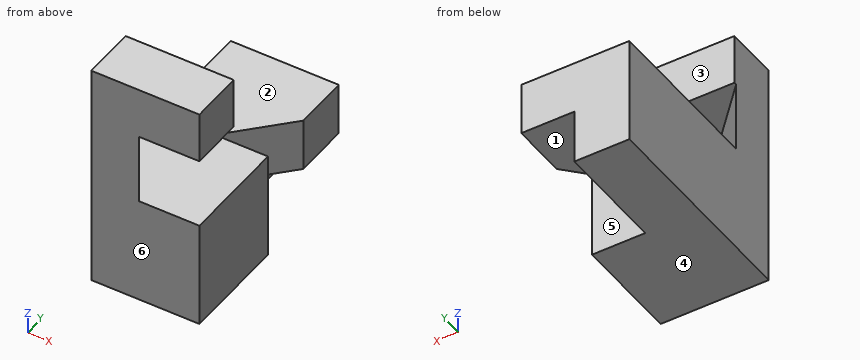
from build123d import *

# Parameters (mm, degrees)
F0_W      = 15.5
F0_H      = 15.5
F1_DEPTH  = 7.747
F3_DEPTH  = 10.16
F4_W      = 15.5
F4_H      = 7.75
F5_DEPTH  = 7.366
F6_W      = 7.874
F6_H      = 15.494
F7_DEPTH  = 16.002
F8_W      = 8.001
F8_H      = 7.62
F9_DEPTH  = 7.62
F11_DEPTH = 7.62


with BuildPart() as f1:
    # F0 (on Top) → F1 (new body, symmetric)
    with BuildSketch(Plane.XY):
        Rectangle(F0_W, F0_H)
    extrude(amount=F1_DEPTH, both=True)

    # F2 (on face) → F3 (join)
    with BuildSketch(Plane.XY.offset(7.747)):
        Polygon((-7.75, -0.384), (-7.75, -7.75), (-0.892, -7.75), align=None)
    extrude(amount=F3_DEPTH)

    # F4 (on face) → F5 (join)
    with BuildSketch(Plane.XY.offset(17.907)):
        with Locations((0, -3.875)):
            Rectangle(F4_W, F4_H)
    extrude(amount=F5_DEPTH)

    # F6 (on face) → F7 (join)
    with BuildSketch(Plane(origin=(0, 7.75, 0), x_dir=(-1, 0, 0), z_dir=(0, 1, 0))):
        with Locations((3.813, 0)):
            Rectangle(F6_W, F6_H)
    extrude(amount=F7_DEPTH)

    # F8 (on face) → F9 (join)
    with BuildSketch(Plane.YZ.offset(0.124)):
        with Locations((19.7515, 3.937)):
            Rectangle(F8_W, F8_H)
    extrude(amount=F9_DEPTH)

    # F10 (on face) → F11 (join)
    with BuildSketch(Plane.XY.offset(7.747)):
        Polygon((0.124, 7.75), (7.744, 15.751), (0.124, 15.751), align=None)
    extrude(amount=-F11_DEPTH)


solid = f1.part
Check sheet for the modelled part. Datum: model origin and axes. Units: mm. Face numbers are marked on the shaded views. A direction names the side the tool comes from. Round coordinates to 2 decimals unless told otherwise and drop trailing zeros. Write each loop counter-clockwise with the first axis right and the second up, starting at its lowest first coordinate (ties: lowest second). Pieces come first, ordered by that corner, then holes. Notation, with made-up numbers: (25.5, 66) - (39.5, 66) arc R26 ccw to (39.5, 105) - close; hole circle Ø3 at (64.25, 42.25). An arc over 180 degrees is marked (long way). Return JSON: item names as keys, results as strings.
Q1. Depth check by flat-ended pin: P1, Ø8, axis at x = -3, z = 23, coming from the +Y side; P2, Ø2.5, axis at x = 5.5, y = 15, coming from the -Z side; P3, Ø6, axis at y = 19, z = 4, coming from the +X side. Enter the tip coordinate at first touch or a pass-through.
Returned:
{"P1": "stops at y = 0", "P2": "stops at z = 0.13", "P3": "stops at x = 7.74"}
Q2. Access from +Z, -Z, +X, -X, +Y, -Y to the whole of each face (thin tool, end or side, straight path). Record for the marked faces 1, 2 and 3.
Returned:
{"face 1": "-Z, +X, +Y", "face 2": "+X, +Y", "face 3": "+Z, +X, -X, +Y"}
Q3. Draft check along Y on the marked faces 4, 5 and 6. Enter one of: released by +Y, released by -Y, zero draft, split by the parting line, or undercut.
Returned:
{"face 4": "zero draft", "face 5": "undercut", "face 6": "released by -Y"}
Q4. Cross-section at B-B (z = 3.5). Record the boundary of the cut face in (x, y), then the cut area to 3 significant figures.
Returned:
{"outline": "(-7.75, -7.75) - (7.75, -7.75) - (7.75, 7.75) - (0.12, 7.75) - (7.74, 15.75) - (7.74, 23.75) - (-7.75, 23.75) - close", "area": "458 mm²"}
Q5. Cross-section at A-A (x = 1). Record the boundary of the cut face in (y, z), then the cut area to 3 significant figures.
Returned:
{"outline": "(-7.75, -7.75) - (7.75, -7.75) - (7.75, 7.75) - (-7.75, 7.75) - close; (-7.75, 17.91) - (0, 17.91) - (0, 25.27) - (-7.75, 25.27) - close; (8.67, 0.13) - (23.75, 0.13) - (23.75, 7.75) - (8.67, 7.75) - close", "area": "412 mm²"}
Q6. Scan lines: L1, parallel to Z at x = -4.5, y = -1; L2, parallel to Z at x = 2.5, y = 20.5; L3, parallel to Z at x = -1, y = 12. Record each from-to range of solid material in increasing order. Write a range as from..to.
Returned:
{"L1": "z = -7.75..7.75, 17.91..25.27", "L2": "z = 0.13..7.75", "L3": "z = -7.75..7.75"}
Q7. Cross-section at D-D (x = -6). Record the boundary of the cut face in (y, z).
Returned:
{"outline": "(-7.75, -7.75) - (23.75, -7.75) - (23.75, 7.75) - (-2.26, 7.75) - (-2.26, 17.91) - (0, 17.91) - (0, 25.27) - (-7.75, 25.27) - close"}
Q8. Cross-section at C-C (y = 20.5). Record the boundary of the cut face in (x, z).
Returned:
{"outline": "(-7.75, -7.75) - (0.12, -7.75) - (0.12, 0.13) - (7.74, 0.13) - (7.74, 7.75) - (-7.75, 7.75) - close"}
